from build123d import *

# Parameters (mm, degrees)
SKETCH1_W           = 15
SKETCH1_H           = 10
BOSS_EXTRUDE1_DEPTH = 180
SKETCH2_W           = 3.8
SKETCH2_H           = 3.8
BOSS_EXTRUDE2_DEPTH = 3.8
SKETCH3_R           = 2.5
CUT_EXTRUDE1_DEPTH  = 2


with BuildPart() as part:
    # Sketch1 → Boss-Extrude1 (new body)
    with BuildSketch(Plane.XY):
        Rectangle(SKETCH1_W, SKETCH1_H)
    extrude(amount=BOSS_EXTRUDE1_DEPTH)

    # Sketch2 → Boss-Extrude2 (add)
    with BuildSketch(Plane.XY.offset(180)):
        Rectangle(SKETCH2_W, SKETCH2_H)
    extrude(amount=BOSS_EXTRUDE2_DEPTH)

    # Sketch3 → Cut-Extrude1 (cut)
    with BuildSketch(Plane(origin=(0, 5, 0), x_dir=(1, 0, 0), z_dir=(0, 1, 0))):
        with Locations((0, -120)):
            Circle(SKETCH3_R)
    extrude(amount=-CUT_EXTRUDE1_DEPTH, mode=Mode.SUBTRACT)


solid = part.part
Can you work these out from the model? Positions are in its coordinate system, mm. A direction names the side the tool comes from. Give positions to 0.01 mm unless a question says otherwise; leave off trailing zeros. Order: outer loops, then holes, each group sorted by start corner. A loop starts at its lowest first (then second) coordinate and runs counter-clockwise, first axis right, second up. Notation, with made-up numbers: M -2.75,45.5 L 55.25,45.5 A27 ccw 55.25,81.5 Z; hole C 32.25,52 d2. An arc over 180 degrees is marked long. Use one line per item in the form item = value. Start each with the question number.
Item 1: We'd pull the mould along Z, two halves only. Please class faces 1 (the flat face through (0, 3, 120)), 2 (the cylindrical face through (-0.33, 4.01, 117.52)), 3 (the flat face through (0, 0, 183.8)), 4 (the flat face through (-7.5, 0, 89)): +Z half, -Z half, draft (parallel to the pull), parting line (faces both ways), or undercut.
Item 2: Will these pins go through, and if not, where does the flat tip stop? pin 1 Ø3 at (y, z) = (0.5, 182) entering from -X; pin 2 Ø4 at (x, z) = (-0.5, 120.5) entering from +Y; pin 3 Ø1.9 at (x, z) = (-0.5, 181.5) entering from +Y; pin 4 Ø1 at (x, y) = (3, -0.5) entering from +Z.
Item 3: If we section it at A-A (x = 0): Write out the boundary of the cut face in (y, z), then the cut area to 3 significant figures.
Item 4: If we section it at B-B (z = 120): Write out the boundary of the cut face in (x, y).
Item 5: For faces 5 (the flat face through (0, 1.9, 182)), 6 (the flat face through (1.9, 0, 182)), 7 (the flat face through (-1.9, 0, 182)), 8 (the flat face through (0, 0, 0)), 9 (the flat face through (0, -1.9, 182)), which set-ups out of +Z, -Z, +X, -X, +Y, -Y let a thin tool reach every point of the face, with its end or its side?
Item 6: If I drill on line 1 along X through (y, z) = (4.55, 120); line 2 along Z through (x, y) = (0, 4.45); line 3 along Z through (x, y) = (3.5, 1.5), over which ranges is the centre line in solid material (lowest first)?
Outcome:
q1.face_1 = undercut
q1.face_2 = undercut
q1.face_3 = +Z half
q1.face_4 = draft
q2.pin_1 = -1.9
q2.pin_2 = 5
q2.pin_3 = 1.9
q2.pin_4 = 180
q3.outline = M -5,0 L 5,0 L 5,117.5 L 3,117.5 L 3,122.5 L 5,122.5 L 5,180 L 1.9,180 L 1.9,183.8 L -1.9,183.8 L -1.9,180 L -5,180 Z
q3.area = 1,800 mm2
q4.outline = M -7.5,-5 L 7.5,-5 L 7.5,5 L 2.5,5 L 2.5,3 L -2.5,3 L -2.5,5 L -7.5,5 Z
q5.face_5 = +Z, +X, -X, +Y
q5.face_6 = +Z, +X, +Y, -Y
q5.face_7 = +Z, -X, +Y, -Y
q5.face_8 = -Z, +X, -X, +Y, -Y
q5.face_9 = +Z, +X, -X, -Y
q6.line_1 = -7.5 to -2.5, 2.5 to 7.5
q6.line_2 = 0 to 117.5, 122.5 to 180
q6.line_3 = 0 to 180
